Design review of the part built by this model. Coordinates are the model's own, in mm. Face numbers are marked on the shaded views. Coordinates: 2 decimals unless noted, no trailing zeros. Write each loop counter-clockwise with the first axis right and the second up, starting at its lowest first coordinate (ties: lowest second). Pieces come first, ordered by that corner, then holes. Notation, with made-up numbers: (-15.75, -16.75) - (18.25, -16.75) arc R16 cw to (18.25, -0.75) - close; hole circle Ø7 at (89.5, 56.25). An arc over 180 degrees is marked (long way). One line per item, written item: value.
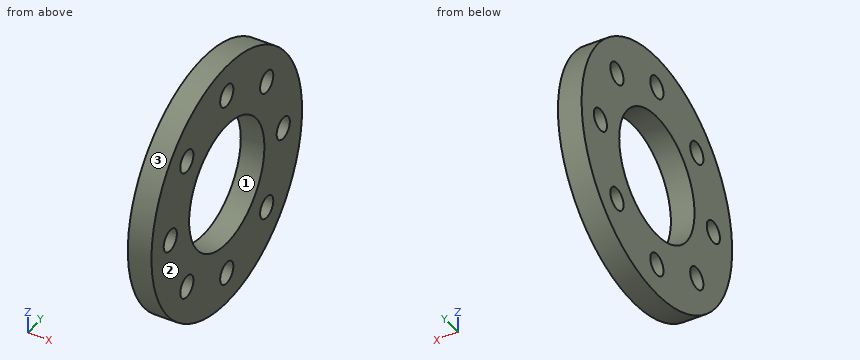
from build123d import *

# Parameters (mm, degrees)
F0_R     = 127
F0_R_2   = 11.1125
F0_R_3   = 63.5
F1_DEPTH = 23.8125


with BuildPart() as f1:
    # F0 (on Right) → F1 (new body)
    with BuildSketch(Plane.YZ):
        Circle(F0_R)
        with Locations((-67.351921, -67.351921)):
            Circle(F0_R_2, mode=Mode.SUBTRACT)
        with Locations((0, -95.25)):
            Circle(F0_R_2, mode=Mode.SUBTRACT)
        with Locations((67.351921, -67.351921)):
            Circle(F0_R_2, mode=Mode.SUBTRACT)
        with Locations((-95.25, 0)):
            Circle(F0_R_2, mode=Mode.SUBTRACT)
        with Locations((-67.351921, 67.351921)):
            Circle(F0_R_2, mode=Mode.SUBTRACT)
        Circle(F0_R_3, mode=Mode.SUBTRACT)
        with Locations((95.25, 0)):
            Circle(F0_R_2, mode=Mode.SUBTRACT)
        with Locations((0, 95.25)):
            Circle(F0_R_2, mode=Mode.SUBTRACT)
        with Locations((67.351921, 67.351921)):
            Circle(F0_R_2, mode=Mode.SUBTRACT)
    extrude(amount=F1_DEPTH)


solid = f1.part
1. Insertion check: pin 1 Ø12 at (x, z) = (12.5, -92) entering from -Y; pin 2 Ø2 at (x, y) = (14.5, -69.5) entering from +Z; pin 3 Ø4 at (x, y) = (11.5, -40.5) entering from -Z; pin 4 Ø1.5 at (y, z) = (-21, -100.5) entering from -X. Each pin has a flat end and moves straight along its axis. Give the tip position at first contact, or say it passes through.
Answer block:
pin 1: stops at y = -93.45
pin 2: stops at z = 106.94
pin 3: stops at z = -121.02
pin 4: stops at x = 0
2. Consider section C-C, the plane y = -29. Write out the cut boundary in (x, z).
Answer block:
outline: (0, -123.64) - (23.81, -123.64) - (23.81, -56.49) - (0, -56.49) - close; (0, 56.49) - (23.81, 56.49) - (23.81, 123.64) - (0, 123.64) - close
3. Consider section D-D, the plane x = 12.25. Give the number of separate pieces and of enclosed holes in the cut face, then the cut area to 3 significant figures.
Answer block:
separate pieces: 1
enclosed holes: 9
area: 34,900 mm^2
4. Consider section A-A, the plane y = 0. Write out the cut boundary in (x, z), then the cut area to 3 significant figures.
Answer block:
outline: (0, -127) - (23.81, -127) - (23.81, -106.36) - (0, -106.36) - close; (0, -84.14) - (23.81, -84.14) - (23.81, -63.5) - (0, -63.5) - close; (0, 63.5) - (23.81, 63.5) - (23.81, 84.14) - (0, 84.14) - close; (0, 106.36) - (23.81, 106.36) - (23.81, 127) - (0, 127) - close
area: 1,970 mm^2
5. Wall thickness on line 1 along Z through (x, y) = (4.5, -0.5); line 2 along Z through (x, y) = (2.25, -73.5); line 3 along Z through (x, y) = (16.5, 67) (3 decimals): over which ranges is each line inside the solid? List them lowest first.
Answer block:
line 1: z = -127 to -106.35, -84.15 to -63.5, 63.5 to 84.15, 106.35 to 127
line 2: z = -103.57 to -76.61, -58.1 to 58.1, 76.61 to 103.57
line 3: z = -107.889 to -78.459, -56.245 to 56.245, 78.459 to 107.889
6. Mouldability with a two-part tool opening along Z and no side actions: class the marked faces 1, 2 and 3 as released by +Z, released by -Z, zero draft, split by the parting line, or undercut.
Answer block:
face 1: undercut
face 2: zero draft
face 3: split by the parting line
